Autodesk Fusion 360 part; units mm, degrees
sketch "スケッチ1" plane through (0, 0, 0) normal (0, 0, 1) x (1, 0, 0)
  line L0 (3, 1.7321) -> (0, 3.4641)
  line L1 (0, 3.4641) -> (-3, 1.7321)
  line L2 (-3, 1.7321) -> (-3, -1.7321)
  line L3 (-3, -1.7321) -> (0, -3.4641)
  line L4 (0, -3.4641) -> (3, -1.7321)
  line L5 (3, -1.7321) -> (3, 1.7321)
  circle A0 centre (0, 0) radius 1.5
extrude "押し出し1" add sketch "スケッチ1" along normal blind 35
sketch "スケッチ2" plane through (0, 0, 35) normal (0, 0, 1) x (-1, 0, 0)
  circle A0 centre (0, 0) radius 1.5
  line L0 (-3, 1.7321) -> (-3, -1.7321)
  line L1 (-3, -1.7321) -> (0, -3.4641)
  line L2 (0, -3.4641) -> (3, -1.7321)
  line L3 (3, -1.7321) -> (3, 1.7321)
  line L4 (3, 1.7321) -> (0, 3.4641)
  line L5 (0, 3.4641) -> (-3, 1.7321)
  line L6 (-3.5, 0) -> (-1.75, -3.0311)
  line L7 (-1.75, -3.0311) -> (1.75, -3.0311)
  line L8 (1.75, -3.0311) -> (3.5, 0)
  line L9 (3.5, 0) -> (1.75, 3.0311)
  line L10 (1.75, 3.0311) -> (-1.75, 3.0311)
  line L11 (-1.75, 3.0311) -> (-3.5, 0)
extrude "押し出し2" add sketch "スケッチ2" along normal blind 4 contours L0 L1 L2 L3 L4 L5 L6 L7 L8 L9 L10 L11 | L0 L6 L11 | L5 L10 L11 | L1 L6 L7 | L4 L9 L10 | L2 L7 L8 | L3 L8 L9
extrude "押し出し3" cut 6 faces at (0, -3.1754, 35) (2.75, -1.5877, 35) (-2.75, -1.5877, 35) (-2.75, 1.5877, 35) (0, 3.1754, 35) (2.75, 1.5877, 35) along direction (0, 0, -1) blind 40
extrude "押し出し4" add 6 faces at (1.5833, 2.7424, 35) (3.1667, 0, 35) (-1.5833, 2.7424, 35) (1.5833, -2.7424, 35) (-1.5833, -2.7424, 35) (-3.1667, 0, 35) along direction (0, 0, -1) blind 35
extrude "押し出し5" cut 1 faces at (2.2005, 1.2273, 39) along direction (0, 0, -1) blind 4
Geometry: final body of the model. Coordinates: model frame, mm. Give positions to 0.01 mm unless a question says otherwise; leave off trailing zeros. Order: outer loops, then holes, each group sorted by start corner. A loop starts at its lowest first (then second) coordinate and runs counter-clockwise, first axis right, second up. Notation, with made-up numbers: (12, 42) -> (55, 42) arc R21 cw to (55, 60) -> close; hole circle Ø11 at (26, -28). An arc over 180 degrees is marked (long way). Answer as a JSON object with one key per item and string values.
Q1. Section C-C (y = 0.75). Output: boundary loops of the cut face in (x, z), plus the area to 3 significant figures.
Entries:
{"outline": "(-3.07, 0) -> (-1.3, 0) -> (-1.3, 35) -> (-3.07, 35) -> close; (1.3, 0) -> (3.07, 0) -> (3.07, 35) -> (1.3, 35) -> close", "area": "124 mm^2"}
Q2. First-contact query: pin 1 (1 mm diameter, centred on y = 1, z = 18.5, fed in from +X). Flat tip, straight axial feed; report the tip coordinate or a pass-through.
Entries:
{"pin 1": "stops at x = 3.21"}
Q3. Draft query along Y for faces 1 (the cylindrical face through (-1.5, -0.07, 17.26)), 2 (the flat face through (2.61, 1.54, 17.74)), 3 (the flat face through (2, 0, 0)). Return one class per face: released by +Y, released by -Y, zero draft, split by the parting line, or undercut.
Entries:
{"face 1": "undercut", "face 2": "released by +Y", "face 3": "zero draft"}
Q4. Section D-D (x = 2.5). Output: boundary loops of the cut face in (y, z), plus the area to 3 significant figures.
Entries:
{"outline": "(-1.73, 0) -> (1.73, 0) -> (1.73, 35) -> (-1.73, 35) -> close", "area": "121 mm^2"}
Q5. Material intervals for probe 1 along Y at (x, z) = (0, 22.5); probe 2 along X at (y, z) = (-1.25, 25.5); probe 3 along X at (y, z) = (-1, 29.5), sorted ascending.
Entries:
{"probe 1": "y = -3.03 to -1.5, 1.5 to 3.03", "probe 2": "x = -2.78 to -0.83, 0.83 to 2.78", "probe 3": "x = -2.92 to -1.12, 1.12 to 2.92"}
Q6. Section A-A (x = 0). Output: boundary loops of the cut face in (y, z).
Entries:
{"outline": "(-3.03, 0) -> (-1.5, 0) -> (-1.5, 35) -> (-3.03, 35) -> close; (1.5, 0) -> (3.03, 0) -> (3.03, 35) -> (1.5, 35) -> close"}
Q7. Section B-B (z = 11). Output: boundary loops of the cut face in (x, y), plus the area to 3 significant figures.
Entries:
{"outline": "(-3.5, 0) -> (-1.75, -3.03) -> (1.75, -3.03) -> (3.5, 0) -> (1.75, 3.03) -> (-1.75, 3.03) -> close; hole circle Ø3 at (0, 0)", "area": "24.8 mm^2"}
